Design review of the part built by this model. Coordinates are the model's own, in mm. Face numbers are marked on the shaded views. A direction names the side the tool comes from. Coordinates: 2 decimals unless noted, no trailing zeros. Loops run counter-clockwise (first coordinate to the right, second up) from the corner with the lowest first, then second, coordinate; pieces in that order, holes last.
Q1. For P1, Ø5.5, axis at x = 0.5, y = 13, coming from the +Z side; P2, Ø10, axis at x = 6.5, z = 3.5, coming from the +Y side; P3, Ø1, axis at x = 11, z = -18.5, coming from the +Y side, all flat-tipped, find the tip position at first contact; note any pin that passes through.
Q2. Add section A-A on x = 6. Give the boundary of the cut face in (y, z).
Q3. Add section B-B on z = 32. Give the boundary of the cut face in (x, y).
Q4. Draft analysis for pull direction Y (two halves, no side actions). For the marked faces 5, 6 and 7, state which applies: released by +Y, released by -Y, zero draft, split by the parting line, or undercut.
Q5. Wall thickness on probe 1 along Y at (x, z) = (20, 17.95); probe 2 along Y at (x, z) = (20, 26.5); probe 3 along Y at (x, z) = (25, -11.5): over which ranges is each line inside the solid? List them lowest first.
Q6. Add section C-C on z = 21. Give the boundary of the cut face in (x, y), and give its area (3 significant figures).
Q7. Machinability: for the marked faces 1, 2, 3 and 4, which of the approach directions +Z, -Z, +X, -X, +Y, -Y give a long, thin tool a straight path to every point of the face, cutting with its end or side? Answer none if there is none.
Autodesk Inventor part; units mm, degrees
ref_plane "Work Plane1" through (0, 0, 2.5) normal (0, 0, 1) x (1, 0, 0)
ref_plane "YZ Plane" through (0, 0, 0) normal (1, 0, 0) x (0, 1, 0)
ref_plane "XZ Plane" through (0, 0, 0) normal (0, 1, 0) x (-1, 0, 0)
sketch "Sketch1" plane through (0, 0, 0) normal (0, 0, 1) x (1, 0, 0)
  line L0 (2.8104, 0) -> (30.1896, 0)
  line L1 (33, 0) -> (33, 27.5) construction
  line L2 (30.1896, 27.5) -> (2.8104, 27.5)
  line L3 (0, 27.5) -> (0, 0) construction
  line L4 (-0.5, 13.75) -> (33.5, 13.75) construction
  arc A0 (-0.1846, 24.6731) -> (-0.1846, 2.8269) centre (188.8125, 13.75) ccw
  arc A1 (33.1846, 2.8269) -> (33.1846, 24.6731) centre (-155.8125, 13.75) ccw
  arc A2 (2.8104, 27.5) -> (-0.1846, 24.6731) centre (2.8104, 24.5) ccw
  arc A3 (33.1846, 24.6731) -> (30.1896, 27.5) centre (30.1896, 24.5) ccw
  arc A4 (-0.1846, 2.8269) -> (2.8104, 0) centre (2.8104, 3) ccw
  arc A5 (30.1896, 0) -> (33.1846, 2.8269) centre (30.1896, 3) ccw
  dimension "d0" = 33
  dimension "d1" = 27.5
  dimension "d2" = 0.5
  dimension "d3" = 0.5
  dimension "d4" = 3
extrude "Extrusion1" add sketch "Sketch1" along normal mid plane 39
ref_plane "Work Plane1" through (0, 0, 2.5) normal (0, 0, 1) x (1, 0, 0)
sketch "Sketch2" plane through (0, 0, 2.5) normal (0, 0, 1) x (1, 0, 0)
  arc A0 (2.8104, 27.5) -> (-0.1846, 24.6731) centre (2.8104, 24.5) ccw
  arc A1 (-0.1846, 24.6731) -> (-0.1846, 2.8269) centre (188.8125, 13.75) ccw
  arc A2 (-0.1846, 2.8269) -> (2.8104, 0) centre (2.8104, 3) ccw
  line L0 (2.8104, 0) -> (30.1896, 0)
  arc A3 (30.1896, 0) -> (33.1846, 2.8269) centre (30.1896, 3) ccw
  arc A4 (33.1846, 2.8269) -> (33.1846, 24.6731) centre (-155.8125, 13.75) ccw
  arc A5 (33.1846, 24.6731) -> (30.1896, 27.5) centre (30.1896, 24.5) ccw
  line L1 (30.1896, 27.5) -> (2.8104, 27.5)
  arc A6 (-0.1846, 24.6731) -> (-0.1846, 2.8269) centre (188.8125, 13.75) ccw
  line L2 (-0.5, 13.75) -> (33.5, 13.75) construction
  arc A7 (-1.3139, 26.3) -> (-1.6821, 24.7596) centre (2.8104, 24.5) ccw
  arc A8 (34.6821, 24.7596) -> (34.3139, 26.3) centre (30.1896, 24.5) ccw
  arc A9 (34.6821, 2.7404) -> (34.6821, 24.7596) centre (-155.8125, 13.75) ccw
  arc A10 (34.3139, 1.2) -> (34.6821, 2.7404) centre (30.1896, 3) ccw
  arc A11 (-1.6821, 2.7404) -> (-1.3139, 1.2) centre (2.8104, 3) ccw
  line L3 (0.5191, 27.5) -> (32.4809, 27.5)
  line L4 (0.5191, 0) -> (32.4809, 0)
  arc A12 (-1.6821, 24.7596) -> (-1.6821, 2.7404) centre (188.8125, 13.75) ccw
  arc A13 (34.3139, 26.3) -> (32.4809, 27.5) centre (32.4809, 25.5) ccw
  arc A14 (0.5191, 27.5) -> (-1.3139, 26.3) centre (0.5191, 25.5) ccw
  arc A15 (-1.3139, 1.2) -> (0.5191, 0) centre (0.5191, 2) ccw
  arc A16 (32.4809, 0) -> (34.3139, 1.2) centre (32.4809, 2) ccw
  point P0 (0, 0)
  point P1 (33.5437, 27.5)
  point P2 (33.5437, 0)
  point P3 (-0.5437, 0)
  point P4 (-0.5437, 27.5)
  dimension "d9" = 1.5
  dimension "d10" = 2
  dimension "d11" = 2
  dimension "d12" = 2
  dimension "d13" = 2
extrude "Extrusion2" add sketch "Sketch2" along normal mid plane 18.5 contours A0 A1 A2 L4 A15 A11 A12 A7 A14 L3 | L3 A13 A8 A9 A10 A16 L4 A3 A4 A5
sketch "Sketch3" plane through (0, 0, 2.5) normal (0, 0, 1) x (1, 0, 0)
  arc A0 (-0.1846, 2.8269) -> (2.8104, 0) centre (2.8104, 3) ccw
  arc A1 (-0.1846, 24.6731) -> (-0.1846, 2.8269) centre (188.8125, 13.75) ccw
  arc A2 (2.8104, 27.5) -> (-0.1846, 24.6731) centre (2.8104, 24.5) ccw
  line L0 (2.8104, 27.5) -> (0.5191, 27.5)
  arc A3 (0.5191, 27.5) -> (-1.3139, 26.3) centre (0.5191, 25.5) ccw
  arc A4 (-1.3139, 26.3) -> (-1.6821, 24.7596) centre (2.8104, 24.5) ccw
  arc A5 (-1.6821, 24.7596) -> (-1.6821, 2.7404) centre (188.8125, 13.75) ccw
  arc A6 (-1.6821, 2.7404) -> (-1.3139, 1.2) centre (2.8104, 3) ccw
  arc A7 (-1.3139, 1.2) -> (0.5191, 0) centre (0.5191, 2) ccw
  line L1 (0.5191, 0) -> (2.8104, 0)
  arc A8 (30.1896, 0) -> (33.1846, 2.8269) centre (30.1896, 3) ccw
  line L2 (30.1896, 0) -> (32.4809, 0)
  arc A9 (32.4809, 0) -> (34.3139, 1.2) centre (32.4809, 2) ccw
  arc A10 (34.3139, 1.2) -> (34.6821, 2.7404) centre (30.1896, 3) ccw
  arc A11 (34.6821, 2.7404) -> (34.6821, 24.7596) centre (-155.8125, 13.75) ccw
  arc A12 (34.6821, 24.7596) -> (34.3139, 26.3) centre (30.1896, 24.5) ccw
  arc A13 (34.3139, 26.3) -> (32.4809, 27.5) centre (32.4809, 25.5) ccw
  line L3 (32.4809, 27.5) -> (30.1896, 27.5)
  arc A14 (33.1846, 24.6731) -> (30.1896, 27.5) centre (30.1896, 24.5) ccw
  arc A15 (33.1846, 2.8269) -> (33.1846, 24.6731) centre (-155.8125, 13.75) ccw
  point P0 (0, 0)
extrude "Extrusion3" cut sketch "Sketch3" along normal mid plane 14.7
sketch "Sketch4" plane through (2.8104, 0, -19.5) normal (0, -1, 0) x (1, 0, 0)
  line L0 (27.3792, 39) -> (0, 39) construction
  line L1 (13.6896, 39) -> (13.6896, 22) construction
  line L2 (13.6896, 22) -> (-8.8104, 22) construction
  line L3 (13.6896, 22) -> (36.1896, 22) construction
  line L4 (9.3896, 51.4625) -> (9.3896, -5.4859) construction
  line L5 (17.1896, 54.9508) -> (17.1896, -9.4609) construction
  line L6 (-8.8104, 31.25) -> (38.6008, 31.25) construction
  point P0 (-2.8104, 19.5)
  dimension "d18" = 17
  dimension "d19" = 22.5
  dimension "d20" = 22.5
  dimension "d21" = 26.8
  dimension "d22" = 7.8
sketch "Sketch5" plane through (2.8104, 27.5, 19.5) normal (0, 1, 0) x (1, 0, 0)
  line L0 (-8.8104, 7.75) -> (38.6008, 7.75) construction
  line L1 (13.6896, 17) -> (36.1896, 17) construction
  line L2 (17.1896, -15.9508) -> (17.1896, 48.4609) construction
  line L3 (9.3896, -12.4625) -> (9.3896, 44.4859) construction
  line L4 (13.6896, 17) -> (-8.8104, 17) construction
  circle A0 centre (9.3896, 7.75) radius 5.5
  circle A1 centre (9.3896, 7.75) radius 4.25
  point P0 (-2.8104, 19.5)
  dimension "d23" = 11
  dimension "d24" = 8.5
extrude "Extrusion4" add sketch "Sketch5" along normal blind 3
sketch "Sketch6" plane through (2.8104, 27.5, 19.5) normal (0, 1, 0) x (1, 0, 0)
  circle A0 centre (9.3896, 7.75) radius 4.25
  point P0 (-2.8104, 19.5)
extrude "Extrusion5" add sketch "Sketch6" along normal blind 13.4
sketch "Sketch7" plane through (12.2, 40.9, 11.75) normal (0, 1, 0) x (1, 0, 0)
  point P0 (-12.2, 11.75)
  point P1 (-0.0229, 0.0053)
hole "Hole1" at (12.1771, 40.9, 11.7447) direction (0, -1, 0) diameter 6 depth 13.4 tip angle 118
sketch "Sketch8" plane through (0, 0, 19.5) normal (0, 0, 1) x (1, 0, 0)
  line L0 (16.45, 40.9) -> (7.95, 40.9) construction
  line L1 (7.95, 30.5) -> (16.45, 30.5) construction
  arc A0 (2.8104, 27.5) -> (-0.1846, 24.6731) centre (2.8104, 24.5) ccw construction
  arc A1 (-0.1846, 24.6731) -> (-0.1846, 2.8269) centre (188.8125, 13.75) ccw construction
  arc A2 (-0.1846, 2.8269) -> (2.8104, 0) centre (2.8104, 3) ccw construction
  line L2 (2.8104, 0) -> (30.1896, 0) construction
  arc A3 (30.1896, 0) -> (33.1846, 2.8269) centre (30.1896, 3) ccw construction
  arc A4 (33.1846, 2.8269) -> (33.1846, 24.6731) centre (-155.8125, 13.75) ccw construction
  arc A5 (33.1846, 24.6731) -> (30.1896, 27.5) centre (30.1896, 24.5) ccw construction
  line L3 (30.1896, 27.5) -> (2.8104, 27.5) construction
  line L4 (-10.3414, 13.75) -> (38.9041, 13.75) construction
  circle A6 centre (20, 13.75) radius 5.5
  line L5 (12.2, 42.7052) -> (12.2, 21.084) construction
  point P0 (0, 0)
  dimension "d36" = 11
  dimension "d37" = 7.8
extrude "Extrusion6" add sketch "Sketch8" along normal blind 4.5
sketch "Sketch9" plane through (20, 13.75, 24) normal (0, 0, 1) x (1, 0, 0)
  circle A0 centre (0, 0) radius 4.2
  point P0 (-20, -13.75)
  dimension "d40" = 8.4
extrude "Extrusion7" add sketch "Sketch9" along normal blind 11.5
sketch "Sketch10" plane through (20, 13.75, 35.5) normal (0, 0, 1) x (1, 0, 0)
  point P0 (-20, -13.75)
  point P1 (0, 0)
hole "Hole2" at (20, 13.75, 35.5) direction (0, 0, -1) diameter 6 depth 13.4 tip angle 118
sketch "Sketch11" plane through (0, 0, 19.5) normal (0, 0, 1) x (1, 0, 0)
  circle A0 centre (20, 13.75) radius 5.5
  arc A1 (2.8104, 27.5) -> (-0.1846, 24.6731) centre (2.8104, 24.5) ccw
  arc A2 (-0.1846, 24.6731) -> (-0.1846, 2.8269) centre (188.8125, 13.75) ccw
  arc A3 (-0.1846, 2.8269) -> (2.8104, 0) centre (2.8104, 3) ccw
  line L0 (2.8104, 0) -> (30.1896, 0)
  arc A4 (30.1896, 0) -> (33.1846, 2.8269) centre (30.1896, 3) ccw
  arc A5 (33.1846, 2.8269) -> (33.1846, 24.6731) centre (-155.8125, 13.75) ccw
  arc A6 (33.1846, 24.6731) -> (30.1896, 27.5) centre (30.1896, 24.5) ccw
  line L1 (30.1896, 27.5) -> (2.8104, 27.5)
  arc A7 (2.8104, 26.5) -> (0.8137, 24.6154) centre (2.8104, 24.5) ccw
  arc A8 (0.8137, 24.6154) -> (0.8137, 2.8846) centre (188.8125, 13.75) ccw
  arc A9 (0.8137, 2.8846) -> (2.8104, 1) centre (2.8104, 3) ccw
  line L2 (2.8104, 1) -> (30.1896, 1)
  arc A10 (30.1896, 1) -> (32.1863, 2.8846) centre (30.1896, 3) ccw
  arc A11 (32.1863, 2.8846) -> (32.1863, 24.6154) centre (-155.8125, 13.75) ccw
  arc A12 (32.1863, 24.6154) -> (30.1896, 26.5) centre (30.1896, 24.5) ccw
  line L3 (30.1896, 26.5) -> (2.8104, 26.5)
  arc A13 (2.8104, 26.3) -> (1.0134, 24.6039) centre (2.8104, 24.5) ccw
  line L4 (2.8104, 26.3) -> (30.1896, 26.3)
  arc A14 (31.9866, 24.6039) -> (30.1896, 26.3) centre (30.1896, 24.5) ccw
  arc A15 (31.9866, 2.8961) -> (31.9866, 24.6039) centre (-155.8125, 13.75) ccw
  arc A16 (30.1896, 1.2) -> (31.9866, 2.8961) centre (30.1896, 3) ccw
  line L5 (30.1896, 1.2) -> (2.8104, 1.2)
  arc A17 (1.0134, 2.8961) -> (2.8104, 1.2) centre (2.8104, 3) ccw
  arc A18 (1.0134, 24.6039) -> (1.0134, 2.8961) centre (188.8125, 13.75) ccw
  line L6 (-3.7926, 13.75) -> (36.6452, 13.75) construction
  point P0 (0, 0)
  dimension "d50" = 1
  dimension "d51" = 0.2
extrude "Extrusion8" cut sketch "Sketch11" against normal blind 2 contours L3 A12 A11 A10 L2 A9 A8 A7
sketch "Sketch12" plane through (0, 0, -19.5) normal (0, 0, -1) x (-1, 0, 0)
  arc A0 (-1.0134, 2.8961) -> (-1.0134, 24.6039) centre (-188.8125, 13.75) ccw
  arc A1 (-2.8104, 1.2) -> (-1.0134, 2.8961) centre (-2.8104, 3) ccw
  line L0 (-2.8104, 1.2) -> (-30.1896, 1.2)
  arc A2 (-31.9866, 2.8961) -> (-30.1896, 1.2) centre (-30.1896, 3) ccw
  arc A3 (-31.9866, 24.6039) -> (-31.9866, 2.8961) centre (155.8125, 13.75) ccw
  arc A4 (-30.1896, 26.3) -> (-31.9866, 24.6039) centre (-30.1896, 24.5) ccw
  line L1 (-30.1896, 26.3) -> (-2.8104, 26.3)
  arc A5 (-1.0134, 24.6039) -> (-2.8104, 26.3) centre (-2.8104, 24.5) ccw
  circle A6 centre (-20, 13.75) radius 5.5
  arc A7 (0.1846, 24.6731) -> (-2.8104, 27.5) centre (-2.8104, 24.5) ccw
  arc A8 (0.1846, 2.8269) -> (0.1846, 24.6731) centre (-188.8125, 13.75) ccw
  arc A9 (-2.8104, 0) -> (0.1846, 2.8269) centre (-2.8104, 3) ccw
  line L2 (-2.8104, 0) -> (-30.1896, 0)
  arc A10 (-33.1846, 2.8269) -> (-30.1896, 0) centre (-30.1896, 3) ccw
  arc A11 (-33.1846, 24.6731) -> (-33.1846, 2.8269) centre (155.8125, 13.75) ccw
  arc A12 (-30.1896, 27.5) -> (-33.1846, 24.6731) centre (-30.1896, 24.5) ccw
  line L3 (-30.1896, 27.5) -> (-2.8104, 27.5)
  arc A13 (-0.8137, 2.8846) -> (-0.8137, 24.6154) centre (-188.8125, 13.75) ccw
  arc A14 (-0.8137, 24.6154) -> (-2.8104, 26.5) centre (-2.8104, 24.5) ccw
  line L4 (-2.8104, 26.5) -> (-30.1896, 26.5)
  arc A15 (-30.1896, 26.5) -> (-32.1863, 24.6154) centre (-30.1896, 24.5) ccw
  arc A16 (-32.1863, 24.6154) -> (-32.1863, 2.8846) centre (155.8125, 13.75) ccw
  arc A17 (-32.1863, 2.8846) -> (-30.1896, 1) centre (-30.1896, 3) ccw
  line L5 (-30.1896, 1) -> (-2.8104, 1)
  arc A18 (-2.8104, 1) -> (-0.8137, 2.8846) centre (-2.8104, 3) ccw
  point P0 (0, 0)
extrude "Extrusion9" cut sketch "Sketch12" against normal blind 2 contours A18 L5 A17 A16 A15 L4 A14 A13
sketch "Sketch13" plane through (2.8104, 27.5, 19.5) normal (0, 1, 0) x (1, 0, 0)
  line L0 (23.9941, 18.8458) -> (2.9639, 18.8458) construction
  line L1 (2.9639, 18.8458) -> (2.9639, 31.9339) construction
  line L2 (2.9639, 31.9339) -> (23.9941, 31.9339) construction
  line L3 (23.9941, 31.9339) -> (23.9941, 18.8458) construction
  point P0 (-2.8104, 19.5)
decal "Decal1"
sketch "Sketch14" plane through (0, 0, 19.5) normal (0, 0, 1) x (1, 0, 0)
  arc A0 (1.0134, 24.6039) -> (1.0134, 2.8961) centre (188.8125, 13.75) ccw
  arc A1 (1.0134, 2.8961) -> (2.8104, 1.2) centre (2.8104, 3) ccw
  line L0 (2.8104, 1.2) -> (30.1896, 1.2)
  arc A2 (30.1896, 1.2) -> (31.9866, 2.8961) centre (30.1896, 3) ccw
  arc A3 (31.9866, 2.8961) -> (31.9866, 24.6039) centre (-155.8125, 13.75) ccw
  arc A4 (31.9866, 24.6039) -> (30.1896, 26.3) centre (30.1896, 24.5) ccw
  line L1 (30.1896, 26.3) -> (2.8104, 26.3)
  arc A5 (2.8104, 26.3) -> (1.0134, 24.6039) centre (2.8104, 24.5) ccw
  circle A6 centre (20, 13.75) radius 5.5
  circle A7 centre (20, 13.75) radius 8.5
  point P0 (0, 0)
  dimension "d81" = 17
extrude "Extrusion10" cut sketch "Sketch14" against normal blind 2 contours A7
properties part number "AD20P-1230A DC Pump"
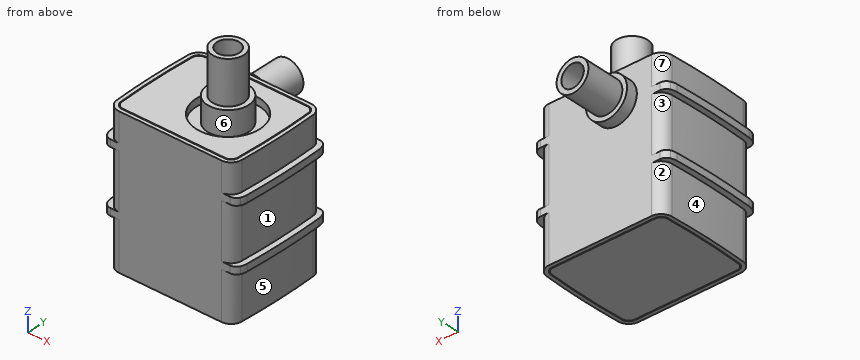
Entries:
1. P1: stops at z = 19.5
1. P2: stops at y = 30.5
1. P3: stops at y = 27.5
2. outline: (0, -19.5) - (1, -19.5) - (1, -17.5) - (1.2, -17.5) - (1.2, -19.5) - (26.3, -19.5) - (26.3, -17.5) - (26.5, -17.5) - (26.5, -19.5) - (27.5, -19.5) - (27.5, 19.5) - (26.5, 19.5) - (26.5, 17.5) - (26.3, 17.5) - (26.3, 19.5) - (1.2, 19.5) - (1.2, 17.5) - (1, 17.5) - (1, 19.5) - (0, 19.5) - close
3. outline: circle Ø8.4 at (20, 13.75); hole circle Ø6 at (20, 13.75)
4. face 5: split by the parting line
4. face 6: undercut
4. face 7: released by +Y
5. probe 1: y = 0 to 1, 1.2 to 5.25, 8.25 to 19.25, 22.25 to 26.3, 26.5 to 27.5
5. probe 2: y = 9.55 to 10.75, 16.75 to 17.95
5. probe 3: y = 0 to 27.5
6. outline: circle Ø11 at (20, 13.75); hole circle Ø2.34 at (20, 13.75)
6. area: 90.7 mm2
7. face 1: +X
7. face 2: -Z, -X, +Y
7. face 3: -X, +Y
7. face 4: -Z, -X
